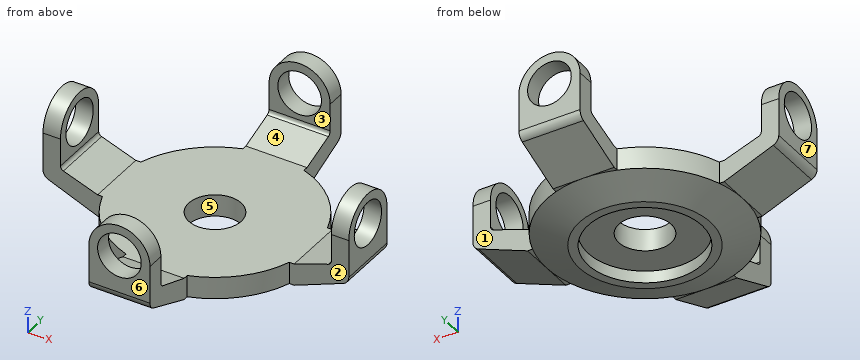
```python
from build123d import *

# Parameters (mm, degrees)
SKETCH3_R                = 22.5
SKETCH3_R_2              = 6
BOSS_EXTRUDE3_DEPTH      = 5
SKETCH4_R                = 15
SKETCH4_R_2              = 13
BOSS_EXTRUDE4_DEPTH      = 2.75
SKETCH10_R               = 7
SKETCH10_R_2             = 5
BOSS_EXTRUDE5_DEPTH      = 2
BOSS_EXTRUDE6_REACH      = 45.9
BOSS_EXTRUDE6_END_RADIUS = 7
SKETCH11_W               = 4
SKETCH11_H               = 14
BOSS_EXTRUDE7_DEPTH      = 14
SKETCH15_W               = 5
SKETCH15_H               = 14
BOSS_EXTRUDE8_DEPTH      = 1.116595
FILLET1_R                = 1
CIRPATTERN4_COUNT        = 4
FILLET1_OF_CIRPATTERN4_R = 1


with BuildPart() as part:
    # Sketch3 → Boss-Extrude3 (new body)
    with BuildSketch(Plane.XY):
        Circle(SKETCH3_R)
        Circle(SKETCH3_R_2, mode=Mode.SUBTRACT)
    extrude(amount=BOSS_EXTRUDE3_DEPTH)

    # Sketch4 → Boss-Extrude4 (add)
    with BuildSketch(Plane(origin=(0, 0, 0), x_dir=(-1, 0, 0), z_dir=(0, 0, -1))):
        with Locations(Location((0, 0, 0), (0, 0, 180))):
            Circle(SKETCH4_R)
        Circle(SKETCH4_R_2, mode=Mode.SUBTRACT)
    extrude(amount=BOSS_EXTRUDE4_DEPTH)

    # Sketch6 → Revolve1 (revolve)
    with BuildSketch(Plane(origin=(0, 0, 0), x_dir=(0, 0, -1), z_dir=(1, 0, 0)), mode=Mode.PRIVATE) as revolve1_sk:
        Polygon((0, 22.5), (0, 15), (2.75, 15), align=None)
    revolve(revolve1_sk.sketch.rotate(Axis((0, 0, 0), (0, 0, -1)), 90), axis=Axis((0, 0, 0), (0, 0, -1)))



with BuildPart() as body_2:
    # Sketch10 → Boss-Extrude5 (new, symmetric)
    with BuildSketch(Plane(origin=(33, 0, 0), x_dir=(0, 0, -1), z_dir=(1, 0, 0))):
        with Locations((-15, 0)):
            Circle(SKETCH10_R)
        with Locations((-15, 0)):
            Circle(SKETCH10_R_2, mode=Mode.SUBTRACT)
    boss_extrude5 = extrude(amount=BOSS_EXTRUDE5_DEPTH, both=True)

    # Boss-Extrude6: up to this cylinder (the profile starts outside it)
    boss_extrude6_end = Plane(origin=(33, 0, 15), z_dir=(-1, 0, 0)) * Cylinder(BOSS_EXTRUDE6_END_RADIUS, 106.8, mode=Mode.PRIVATE)
    # Sketch11 → Boss-Extrude6 (add, up to the surface)
    with BuildSketch(Plane(origin=(0, 0, 8), x_dir=(-1, 0, 0), z_dir=(0, 0, -1)), mode=Mode.PRIVATE) as boss_extrude6_sk1:
        with Locations((-33, 0)):
            Rectangle(SKETCH11_W, SKETCH11_H)
    boss_extrude6_tool1 = extrude(boss_extrude6_sk1.sketch, amount=-BOSS_EXTRUDE6_REACH, mode=Mode.PRIVATE) - boss_extrude6_end
    boss_extrude6 = boss_extrude6_tool1.solids().sort_by_distance((33, 0, 8))[0] + boss_extrude6_tool1.solids().sort_by_distance((33, 0, 8))[1]
    add(boss_extrude6)

    # Sketch12 → Boss-Extrude7 (add)
    with BuildSketch(Plane(origin=(0, -7, 0), x_dir=(1, 0, 0), z_dir=(0, 1, 0))):
        with BuildLine():
            Line((31, -8), (22.5, -5))
            Line((22.5, -5), (22.5, 0))
            Line((22.5, 0), (33.742781353, -4.497112541))
            ThreePointArc((33.742781353, -4.497112541), (34.656134461, -5.232808304), (35, -6.354065923))
            Line((35, -6.354065923), (35, -8))
            Line((35, -8), (31, -8))
        make_face()
    boss_extrude7 = extrude(amount=BOSS_EXTRUDE7_DEPTH)


with BuildPart() as part_1:
    add(part.part)

    add(body_2.part)  # Boss-Extrude8 merges body 2
    # Sketch15 → Boss-Extrude8 (add)
    with BuildSketch(Plane.ZY.offset(-22.5)):
        with Locations((2.5, 0)):
            Rectangle(SKETCH15_W, SKETCH15_H)
    boss_extrude8 = extrude(amount=BOSS_EXTRUDE8_DEPTH)

    # Fillet1
    fillet1_edges = [part_1.edges().sort_by_distance(p)[0] for p in [
        (31, 0, 8),
    ]]
    fillet(fillet1_edges, radius=FILLET1_R)

    # CirPattern4: Boss-Extrude5, Boss-Extrude6, Boss-Extrude7, Boss-Extrude8 ×4 about axis
    cirpattern4_axis = Axis((0, 0, 0), (0, 0, 1))
    add([boss_extrude5.rotate(cirpattern4_axis, i * 360 / CIRPATTERN4_COUNT) for i in range(1, CIRPATTERN4_COUNT)])
    add([boss_extrude6.rotate(cirpattern4_axis, i * 360 / CIRPATTERN4_COUNT) for i in range(1, CIRPATTERN4_COUNT)])
    add([boss_extrude7.rotate(cirpattern4_axis, i * 360 / CIRPATTERN4_COUNT) for i in range(1, CIRPATTERN4_COUNT)])
    add([boss_extrude8.rotate(cirpattern4_axis, i * 360 / CIRPATTERN4_COUNT) for i in range(1, CIRPATTERN4_COUNT)])

    # Fillet1 of CirPattern4
    fillet1_of_cirpattern4_edges = [part_1.edges().sort_by_distance(p)[0] for p in [
        (0, 31, 8),
        (-31, 0, 8),
        (0, -31, 8),
    ]]
    fillet(fillet1_of_cirpattern4_edges, radius=FILLET1_OF_CIRPATTERN4_R)


solid = part_1.part
```
Source: CAD feature listing. Evaluate the final solid. Frame: model axes, mm. Face numbers are marked on the shaded views. A direction names the side the tool comes from. Give positions to 0.01 mm unless a question says otherwise; leave off trailing zeros. Loops run counter-clockwise (first coordinate to the right, second up) from the corner with the lowest first, then second, coordinate; pieces in that order, holes last. Notation, with made-up numbers: (80, 33.25) - (139, 33.25) arc R17 ccw to (139, 63.25) - close; hole circle Ø10 at (30, 25). An arc over 180 degrees is marked (long way). Use CSV: the item, a comma, the result in double quotes.
1) Line query: line 1 (X direction, y = -33.15, z = 15); line 2 (Z direction, x = -1, y = -12); line 3 (X direction, y = -26.5, z = 5.5). Output: solid intervals per line, ascending.
Worked out:
line 1,"x = -7 to -5, 5 to 7"
line 2,"z = 0 to 5"
line 3,"x = -7 to 7"
2) Mould query, pull axis Y, two halves, no side actions, for the marked faces 4, 5, 6 and 7. Classes: +Y half, -Y half, draft (parallel to the pull), parting line (faces both ways), or undercut.
Worked out:
face 4,"undercut"
face 5,"undercut"
face 6,"-Y half"
face 7,"draft"
3) Pin query (flat end, axial travel): P1, Ø0.6, axis at x = 22, y = -4, coming from the -Z side; P2, Ø12, axis at x = -6.5, y = -24.5, coming from the -Z side; P3, Ø1.2, axis at x = -2, y = 22, coming from the -Z side. Return the tip coordinate at first contact, or that it passes through.
Worked out:
P1,"stops at z = -0.16"
P2,"stops at z = -1.16"
P3,"stops at z = -0.37"
4) Cut plane A-A (z = 17). Count the separate pieces of the cut face and the enclosed holes in it, and give its area (3 significant figures).
Worked out:
separate pieces,"8"
enclosed holes,"0"
area,"68.0 mm^2"
5) Cut plane D-D (y = 25.5). Output: boundary loops of the cut face in (x, z).
Worked out:
outline,"(-7, 1.2) - (7, 1.2) - (7, 6.06) - (-7, 6.06) - close"
6) Set-up query: the marked faces 1, 2 and 3. Return all of +Z, -Z, +X, -X, +Y, -Y with unobstructed straight access to the full face (end or side cutting, diameter ignored); none if empty.
Worked out:
face 1,"+Z, -Z, +X, +Y"
face 2,"+Z, -Z, +X, -Y"
face 3,"+Z, +X, -X"
